Autodesk Inventor part; units mm, degrees
ref_plane "YZ Plane" through (0, 0, 0) normal (1, 0, 0) x (0, 1, 0)
ref_plane "XZ Plane" through (0, 0, 0) normal (0, 1, 0) x (-1, 0, 0)
ref_plane "XY Plane" through (0, 0, 0) normal (0, 0, 1) x (1, 0, 0)
sketch "Sketch1" plane through (0, 0, 0) normal (0, 0, 1) x (1, 0, 0)
  circle A0 centre (0, 0) radius 60
  line L0 (-117.4264, -75) -> (-117.4264, 75)
  line L1 (-117.4264, 75) -> (-75, 117.4264)
  line L2 (-75, 117.4264) -> (75, 117.4264)
  line L3 (75, 117.4264) -> (117.4264, 75)
  line L4 (117.4264, 75) -> (117.4264, -75)
  line L5 (117.4264, -75) -> (75, -117.4264)
  line L6 (75, -117.4264) -> (-75, -117.4264)
  line L7 (-75, -117.4264) -> (-117.4264, -75)
  point P0 (-117.4264, 0)
  point P1 (117.4264, 0)
  point P2 (0, 117.4264)
  point P3 (0, -117.4264)
  dimension "d2" = 3
  dimension "d22" = 120
  dimension "d33" = 150
  dimension "d35" = 60
extrude "Plate1" add sketch "Sketch1" along normal blind 3
sketch "Sketch6" plane through (0, 0, 3) normal (0, 0, 1) x (1, 0, 0)
  circle A0 centre (0, 0) radius 65 construction
  circle A1 centre (65, 0) radius 2.75
  dimension "d2" = 3
  dimension "d36" = 130
  dimension "d37" = 5.5
extrude "Cut2" cut sketch "Sketch6" against normal blind 3
pattern_circular "Circular Pattern2" count 8 over 360 about axis through (0, 0, -10) along (0, 0, 1) of "Cut2"
equation "\"d2\" = Thickness"
equation "\"d33\" = Wall_1_width"
equation "\"d35\" = Wall_2_width"
equation "\"d38\" = Thickness"
equation "\"BendReliefWidth\" = Thickness"
equation "\"BendReliefDepth\" = 0.5 * Thickness"
equation "\"CornerReliefSize\" = 4 * Thickness"
equation "\"MinimumRemnant\" = 2 * Thickness"
equation "\"TransitionRadius\" = BendRadius"
equation "\"JacobiRadiusSize\" = BendRadius"
equation "\"GapSize\" = Thickness"
properties part number "TKS 3555 BOTTOM DS cup" material "Stainless Steel"
Geometry check sheet. Reference: the model listing, model coordinates, mm. Give positions to 0.01 mm unless a question says otherwise; leave off trailing zeros. Write each loop counter-clockwise with the first axis right and the second up, starting at its lowest first coordinate (ties: lowest second). Pieces come first, ordered by that corner, then holes.
1) Release check for a two-part mould opening along Y. For faces 1 (the face through (0.121, -62.253, 1.521)), 2 (the face through (-43.642, 47.439, 1.521)), 3 (the face through (96.51, -95.916, 1.479)), 4 (the face through (-96.51, 95.916, 1.479)) record: released by +Y, released by -Y, zero draft, split by the parting line, or undercut.
Values follow:
face 1: undercut
face 2: undercut
face 3: released by -Y
face 4: released by +Y
2) Thickness scan on line 1 (X direction, y = -0.5, z = 2.45); line 2 (X direction, y = -65, z = 1.6); line 3 (X direction, y = -28, z = 2.05). Record the ranges inside material, lowest first.
Values follow:
line 1: x = -117.43 to -67.7, -62.3 to -60, 60 to 62.3, 67.7 to 117.43
line 2: x = -117.43 to -2.75, 2.75 to 117.43
line 3: x = -117.43 to -53.07, 53.07 to 117.43
3) Cross-section at A-A (x = 65). Record the boundary of the cut face in (y, z), plus the area to 3 significant figures.
Values follow:
outline: (-117.43, 0) - (-2.75, 0) - (-2.75, 3) - (-117.43, 3) - close; (2.75, 0) - (117.43, 0) - (117.43, 3) - (2.75, 3) - close
area: 688 mm2
4) Cross-section at C-C (x = 0). Record the boundary of the cut face in (y, z), plus the area to 3 significant figures.
Values follow:
outline: (-117.43, 0) - (-67.75, 0) - (-67.75, 3) - (-117.43, 3) - close; (-62.25, 0) - (-60, 0) - (-60, 3) - (-62.25, 3) - close; (60, 0) - (62.25, 0) - (62.25, 3) - (60, 3) - close; (67.75, 0) - (117.43, 0) - (117.43, 3) - (67.75, 3) - close
area: 312 mm2
